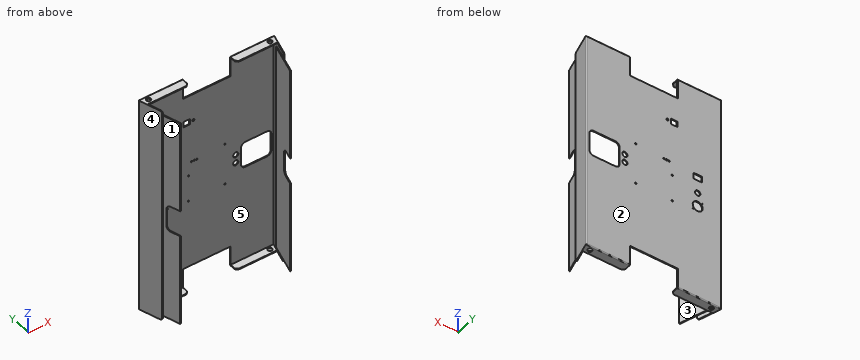
```python
from build123d import *

# Parameters (mm, degrees)
EXTRUSION1_DEPTH             = 500
CONG_1_R                     = 5
EXTRUSION2_DEPTH             = 2
ENL_V_MAT_EXTRU_1_DEPTH      = 2
EXTRUSION3_DEPTH             = 2
ESQUISSE6_W                  = 110
ESQUISSE6_H                  = 46
ENL_V_MAT_EXTRU_7_DEPTH      = 532.648435432
CHANFREIN1_SIZE              = 5
CHANFREIN1_OF_SYM_TRIE4_SIZE = 5
CONG_4_START                 = -157
CONG_4_DEPTH                 = 314
ESQUISSE7_R                  = 5
ENL_V_MAT_EXTRU_8_DEPTH      = 532.648435555
ESQUISSE8_R                  = 6.25
ESQUISSE8_R_2                = 11.5
ESQUISSE8_R_3                = 1
ESQUISSE8_R_4                = 6
ESQUISSE8_R_5                = 2.5
ESQUISSE8_W                  = 20
ESQUISSE8_H                  = 14
ESQUISSE8_W_2                = 15
ESQUISSE8_H_2                = 13
ENL_V_MAT_EXTRU_9_DEPTH      = 2
ESQUISSE9_R                  = 1.6
ESQUISSE9_R_2                = 1.75
ENL_V_MAT_EXTRU_10_DEPTH     = 2


with BuildPart() as part:
    # Esquisse1 → Extrusion1 (new body)
    with BuildSketch(Plane.XY):
        with BuildLine():
            Line((-153.951793051, 0), (153.951793051, 0))
            ThreePointArc((153.951793051, 0), (155.552163839, -0.800494544), (155.871446543, -2.561186662))
            Line((155.871446543, -2.561186662), (141, -53.432004207))
            Line((141, -53.432004207), (139.080346508, -52.870817545))
            Line((139.080346508, -52.870817545), (153.951793051, -2))
            Line((153.951793051, -2), (-153.951793051, -2))
            Line((-153.951793051, -2), (-139.080346508, -52.870817545))
            Line((-139.080346508, -52.870817545), (-141, -53.432004207))
            Line((-141, -53.432004207), (-155.871446543, -2.561186662))
            ThreePointArc((-155.871446543, -2.561186662), (-155.552163839, -0.800494544), (-153.951793051, 0))
        make_face()
    extrude(amount=EXTRUSION1_DEPTH)

    # Congé1
    cong_1_edges = [part.edges().sort_by_distance(p)[0] for p in [
        (-140.040173254, -53.151410876, 0),
        (-140.040173254, -53.151410876, 500),
        (140.040173254, -53.151410876, 500),
        (140.040173254, -53.151410876, 0),
    ]]
    fillet(cong_1_edges, radius=CONG_1_R)

    # Esquisse2 → Extrusion2 (add)
    with BuildSketch(Plane(origin=(-142.369407398, -41.619913609, 0), x_dir=(0, 0, -1), z_dir=(0.9598267461373389, 0.2805933309959605, 0))):
        with BuildLine():
            Line((-490, 23.278192933), (-10, 23.278192933))
            Line((-10, 23.278192933), (-10, -51.721807067))
            Line((-10, -51.721807067), (-220, -51.721807067))
            Line((-220, -51.721807067), (-220, -29.721807067))
            ThreePointArc((-220, -29.721807067), (-222.928932188, -22.650739256), (-230, -19.721807067))
            Line((-230, -19.721807067), (-270, -19.721807067))
            ThreePointArc((-270, -19.721807067), (-277.071067812, -22.650739256), (-280, -29.721807067))
            Line((-280, -29.721807067), (-280, -51.721807067))
            Line((-280, -51.721807067), (-490, -51.721807067))
            Line((-490, -51.721807067), (-490, 23.278192933))
        make_face()
    extrusion2 = extrude(amount=EXTRUSION2_DEPTH)

    # Symétrie1: Extrusion2 across plane
    add(extrusion2.mirror(Plane(origin=(0, 0, 0), x_dir=(0, 0, 1), z_dir=(1, 0, 0))))

    # Esquisse3 → Enlèv. mat.-Extru.1 (cut)
    with BuildSketch(Plane(origin=(0, 0, 0), x_dir=(-1, 0, 0), z_dir=(0, 1, 0))):
        with BuildLine():
            Line((-138.951793051, 220), (-88.951793051, 220))
            ThreePointArc((-88.951793051, 220), (-81.880725239, 222.928932188), (-78.951793051, 230))
            Line((-78.951793051, 230), (-78.951793051, 270))
            ThreePointArc((-78.951793051, 270), (-81.880725239, 277.071067812), (-88.951793051, 280))
            Line((-88.951793051, 280), (-138.951793051, 280))
            ThreePointArc((-138.951793051, 280), (-146.022860862, 277.071067812), (-148.951793051, 270))
            Line((-148.951793051, 270), (-148.951793051, 230))
            ThreePointArc((-148.951793051, 230), (-146.022860862, 222.928932188), (-138.951793051, 220))
        make_face()
    extrude(amount=-ENL_V_MAT_EXTRU_1_DEPTH, mode=Mode.SUBTRACT)

    # Esquisse4 → Extrusion3 (add)
    with BuildSketch(Plane(origin=(0, 0, 0), x_dir=(-1, 0, 0), z_dir=(0, 0, -1))):
        Polygon((153.951793051, -2), (-153.951793051, -2), (-148.689718433, -20), (148.689718433, -20), align=None)
    extrusion3 = extrude(amount=-EXTRUSION3_DEPTH)

    # Esquisse6 → Enlèv. mat.-Extru.7 (cut, through all)
    with BuildSketch(Plane(origin=(0, 0, 0), x_dir=(-1, 0, 0), z_dir=(0, 1, 0))):
        with Locations((0, 23)):
            Rectangle(ESQUISSE6_W, ESQUISSE6_H)
    enl_v_mat_extru_7 = extrude(amount=-ENL_V_MAT_EXTRU_7_DEPTH, mode=Mode.SUBTRACT)

    # Chanfrein1
    chanfrein1_edges = [part.edges().sort_by_distance(p)[0] for p in [
        (55, -20, 1),
        (-55, -20, 1),
    ]]
    chamfer(chanfrein1_edges, length=CHANFREIN1_SIZE)

    # Symétrie4: Extrusion3, Enlèv. mat.-Extru.7 across plane
    add(extrusion3.mirror(Plane.XY.offset(250)))
    add(enl_v_mat_extru_7.mirror(Plane.XY.offset(250)), mode=Mode.SUBTRACT)

    # Chanfrein1 of Symétrie4
    chanfrein1_of_sym_trie4_edges = [part.edges().sort_by_distance(p)[0] for p in [
        (55, -20, 499),
        (-55, -20, 499),
    ]]
    chamfer(chanfrein1_of_sym_trie4_edges, length=CHANFREIN1_OF_SYM_TRIE4_SIZE)

    # Congé4: read off the stored shape, not the designer's step
    # Congé4 outline → Congé4 (cut)
    with BuildSketch(Plane.YZ.offset(CONG_4_START)):
        with BuildLine():
            Line((0, 500), (-2, 500))
            ThreePointArc((-2, 500), (-0.585786438, 499.414213562), (0, 498))
            Line((0, 498), (0, 500))
        make_face()
        with BuildLine():
            Line((0, 0), (0, 2))
            ThreePointArc((0, 2), (-0.585786438, 0.585786438), (-2, 0))
            Line((-2, 0), (0, 0))
        make_face()
    extrude(amount=CONG_4_DEPTH, mode=Mode.SUBTRACT)

    # Esquisse7 → Enlèv. mat.-Extru.8 (cut, through all)
    with BuildSketch(Plane.XY.offset(500)):
        with Locations((-140, -10)):
            Circle(ESQUISSE7_R)
        with Locations((140, -10)):
            Circle(ESQUISSE7_R)
    extrude(amount=-ENL_V_MAT_EXTRU_8_DEPTH, mode=Mode.SUBTRACT)

    # Esquisse8 → Enlèv. mat.-Extru.9 (cut)
    with BuildSketch(Plane(origin=(0, 0, 0), x_dir=(-1, 0, 0), z_dir=(0, 1, 0))):
        with Locations(Location((100.951793051, 250, 0), (0, 0, 90))):
            Circle(ESQUISSE8_R)
        with Locations(Location((100.951793051, 218, 0), (0, 0, 90))):
            Circle(ESQUISSE8_R_2)
        with Locations(Location((111.558394768, 228.606601718, 0), (0, 0, 90))):
            Circle(ESQUISSE8_R_3)
        with Locations(Location((90.345191333, 207.393398282, 0), (0, 0, 90))):
            Circle(ESQUISSE8_R_3)
        with Locations(Location((-66.951793051, 240.5, 0), (0, 0, 90))):
            Circle(ESQUISSE8_R_4)
        with Locations(Location((-66.951793051, 259.5, 0), (0, 0, 90))):
            Circle(ESQUISSE8_R_4)
        with Locations(Location((30.951793051, 391.5, 0), (0, 0, 90))):
            Circle(ESQUISSE8_R_5)
        with Locations((100.951793051, 287)):
            Rectangle(ESQUISSE8_W, ESQUISSE8_H)
        with Locations((46.451793051, 391.5)):
            Rectangle(ESQUISSE8_W_2, ESQUISSE8_H_2)
    extrude(amount=-ENL_V_MAT_EXTRU_9_DEPTH, mode=Mode.SUBTRACT)

    # Esquisse9 → Enlèv. mat.-Extru.10 (cut)
    with BuildSketch(Plane(origin=(0, 0, 0), x_dir=(-1, 0, 0), z_dir=(0, 1, 0))):
        with Locations(Location((-42, 202.5, 0), (0, 0, 90))):
            Circle(ESQUISSE9_R)
        with Locations(Location((-42, 297.5, 0), (0, 0, 90))):
            Circle(ESQUISSE9_R)
        with Locations(Location((42, 202.5, 0), (0, 0, 90))):
            Circle(ESQUISSE9_R)
        with Locations(Location((42, 263.5, 0), (0, 0, 90))):
            Circle(ESQUISSE9_R)
        with Locations(Location((23, 294, 0), (0, 0, 90))):
            Circle(ESQUISSE9_R_2)
        with Locations(Location((29, 294, 0), (0, 0, 90))):
            Circle(ESQUISSE9_R_2)
        with Locations(Location((35, 294, 0), (0, 0, 90))):
            Circle(ESQUISSE9_R_2)
    extrude(amount=-ENL_V_MAT_EXTRU_10_DEPTH, mode=Mode.SUBTRACT)


solid = part.part
```
Geometry check sheet. Reference: the model listing, model coordinates, mm. Face numbers are marked on the shaded views. A direction names the side the tool comes from. Coordinates: 2 decimals unless noted, no trailing zeros. Order: outer loops, then holes, each group sorted by start corner. A loop starts at its lowest first (then second) coordinate and runs counter-clockwise, first axis right, second up.
Item 1: Section check A-A (z = 127.5). Enter the section's corners in (x, y).
Item 2: Tool access check on the marked faces 4 and 5. Record the directions out of +Z, -Z, +X, -X, +Y, -Y that give a thin tool (end or side, any length) a straight path to the whole face; none if there is none.
Item 3: Section check B-B (y = -10). Count the separate pieces of the cut face and the enclosed holes in it, plus the area to 3 significant figures.
Item 4: Section check C-C (x = 49). Enter the section's corners in (y, z).
Item 5: Depth check by flat-ended pin: pin 1 (1.5 mm diameter, centred on x = -55, z = 356, fed in from +Y); pin 2 (14.5 mm diameter, centred on x = -100.95, z = 250, fed in from -Y); pin 3 (2 mm diameter, centred on x = 87, z = 499, fed in from -Y); pin 4 (11 mm diameter, centred on x = 66.95, z = 259.5, fed in from +Y) (3 decimals). Enter the tip coordinate at first touch or a pass-through.
Item 6: Mould release check, pull along Y, two halves, no side actions. Record for the marked faces 1, 2 and 3: released by +Y, released by -Y, zero draft, split by the parting line, or undercut.
Item 7: Scan lines: line 1 along X through (y, z) = (-1.3, 202.5); line 2 along Z through (x, y) = (134, -69.5); line 3 along Y through (x, z) = (-37, 273). Record each from-to range of solid material in increasing order.
Check sheet entries:
1. outline: (-155.87, -2.56) - (-141, -53.43) - (-139.08, -52.87) - (-127.86, -91.26) - (-125.94, -90.7) - (-146.98, -18.72) - (-148.9, -19.28) - (-153.95, -2) - (153.95, -2) - (148.9, -19.28) - (146.98, -18.72) - (125.94, -90.7) - (127.86, -91.26) - (139.08, -52.87) - (141, -53.43) - (155.87, -2.56) arc R2 ccw to (153.95, 0) - (-153.95, 0) arc R2 ccw to start
2. face 4: +Z, -Z, -X, -Y
2. face 5: none
3. separate pieces: 6
3. enclosed holes: 0
3. area: 2,780 mm2
4. outline: (-2, 46) - (0, 46) - (0, 454) - (-2, 454) - close
5. pin 1: stops at y = 0
5. pin 2: stops at y = -2
5. pin 3: stops at y = -20
5. pin 4: passes through
6. face 1: released by -Y
6. face 2: released by +Y
6. face 3: undercut
7. line 1: x = -155.83 to -43.6, -40.4 to 40.4, 43.6 to 155.83
7. line 2: z = 10 to 220.02, 279.98 to 490
7. line 3: y = -2 to 0
